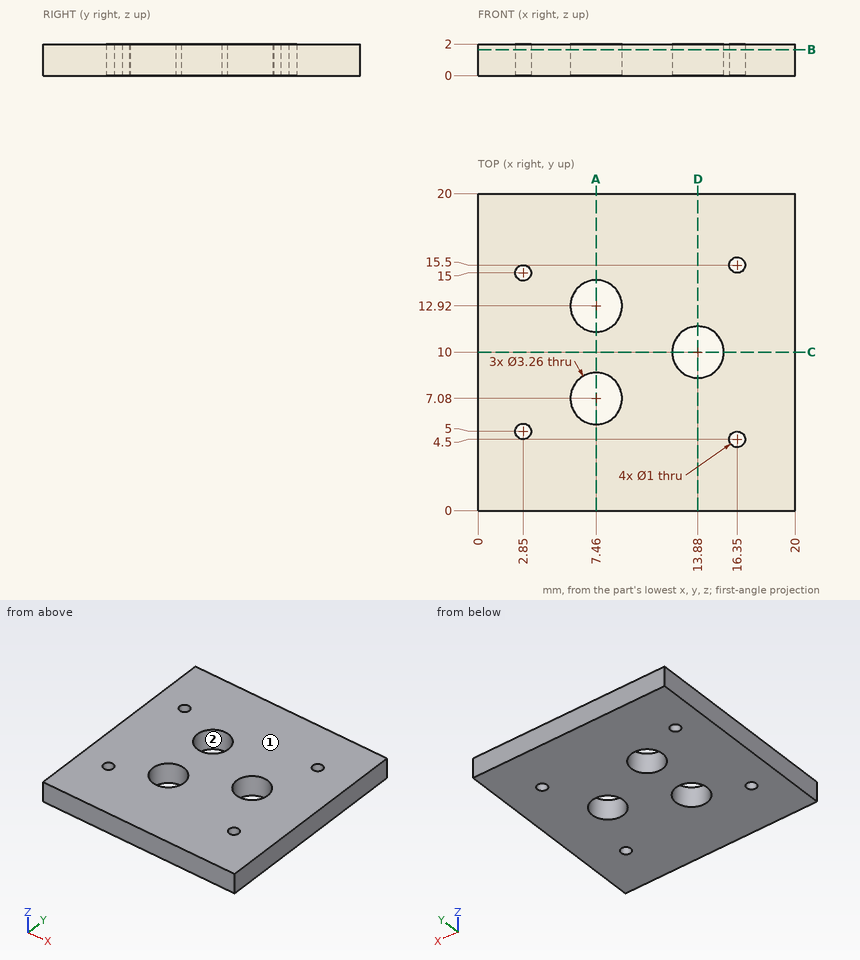
Check sheet for the drawn part. Datum: minimum x, y, z corner. Units: mm. Round coordinates to 2 decimals unless told otherwise and drop trailing zeros. Order: outer loops, then holes, each group sorted by start corner. A loop starts at its lowest first (then second) coordinate and runs counter-clockwise, first axis right, second up. Notation, with made-up numbers: (48.5, -13.75) -> (79.5, -13.75) arc R14 ccw to (79.5, -1.75) -> close; hole circle Ø5 at (-39, 12). An arc over 180 degrees is marked (long way). Put each result on its own line as item: value. Start each with the question number.
(1) Draft check along X on the marked faces 1 and 2. Enter one of: +X half, -X half, draft (parallel to the pull), parting line (faces both ways), or undercut.
(2) Material ranges on line 1 along Y through (x, z) = (16.35, 1.15); line 2 along Y through (x, z) = (2.85, 0.95); line 3 along X through (y, z) = (13, 1.6), recorded low to high.
(3) Section check C-C (y = 10). Enter the section's corners in (x, z), then the cut area to 3 significant figures.
(4) Section check A-A (x = 7.46). Enter the section's corners in (y, z).
(5) Section check D-D (x = 13.88). Enter the section's corners in (y, z), then the cut area to 3 significant figures.
(6) Section check B-B (z = 1.65). Enter the section's corners in (x, y).
Completed:
1. face 1: draft
1. face 2: undercut
2. line 1: y = 0 to 4, 5 to 15, 16 to 20
2. line 2: y = 0 to 4.5, 5.5 to 14.5, 15.5 to 20
2. line 3: x = 0 to 5.83, 9.09 to 20
3. outline: (0, 0) -> (12.25, 0) -> (12.25, 2) -> (0, 2) -> close; (15.51, 0) -> (20, 0) -> (20, 2) -> (15.51, 2) -> close
3. area: 33.5 mm2
4. outline: (0, 0) -> (5.45, 0) -> (5.45, 2) -> (0, 2) -> close; (8.71, 0) -> (11.29, 0) -> (11.29, 2) -> (8.71, 2) -> close; (14.55, 0) -> (20, 0) -> (20, 2) -> (14.55, 2) -> close
5. outline: (0, 0) -> (8.37, 0) -> (8.37, 2) -> (0, 2) -> close; (11.63, 0) -> (20, 0) -> (20, 2) -> (11.63, 2) -> close
5. area: 33.5 mm2
6. outline: (0, 0) -> (20, 0) -> (20, 20) -> (0, 20) -> close; hole circle Ø1 at (2.85, 5); hole circle Ø1 at (2.85, 15); hole circle Ø3.26 at (7.46, 7.08); hole circle Ø3.26 at (7.46, 12.92); hole circle Ø3.26 at (13.88, 10); hole circle Ø1 at (16.35, 4.5); hole circle Ø1 at (16.35, 15.5)
